Geometry: see drawing. Coordinates: mm, zero at the bounding-box minimum. A direction names the side the tool comes from. Round coordinates to 2 decimals unless told otherwise and drop trailing zeros. Loops run counter-clockwise (first coordinate to the right, second up) from the corner with the lowest first, then second, coordinate; pieces in that order, holes last.
(1) Cut plane C-C, the plane y = 3.75. Output: boundary loops of the cut face in (x, z).
(2) Cut plane D-D, the plane x = 21. Output: boundary loops of the cut face in (y, z), and give its area (3 significant figures).
(3) Cut plane B-B, the plane z = 2.5. Output: boundary loops of the cut face in (x, y), and give its area (3 significant figures).
(4) Cut plane A-A, the plane x = 34. Output: boundary loops of the cut face in (y, z).
(5) Draft query along Y for the marked faces 4, 5 and 6. Return one class per face: released by +Y, released by -Y, zero draft, split by the parting line, or undercut.
(6) Access query for the marked faces 1, 2 and 3. Directions: +Z, -Z, +X, -X, +Y, -Y. A direction counts if a zero-diameter tool reaches every point of the face in a straight line with its end or side. Return the directions, or none.
(7) Line query: line 1 (Y direction, x = 30.5, z = 7.25); line 2 (X direction, y = 2.25, z = 9); line 3 (Y direction, x = 4.5, z = 7.5). Output: solid intervals per line, ascending.
(8) First-contact query: pin 1 Ø5 at (x, z) = (19.5, 5) entering from -Y; pin 2 Ø0.9 at (y, z) = (3.5, 6.5) entering from +X. Flat tips, straight axial feed; report the tip coordinate or a pass-through.
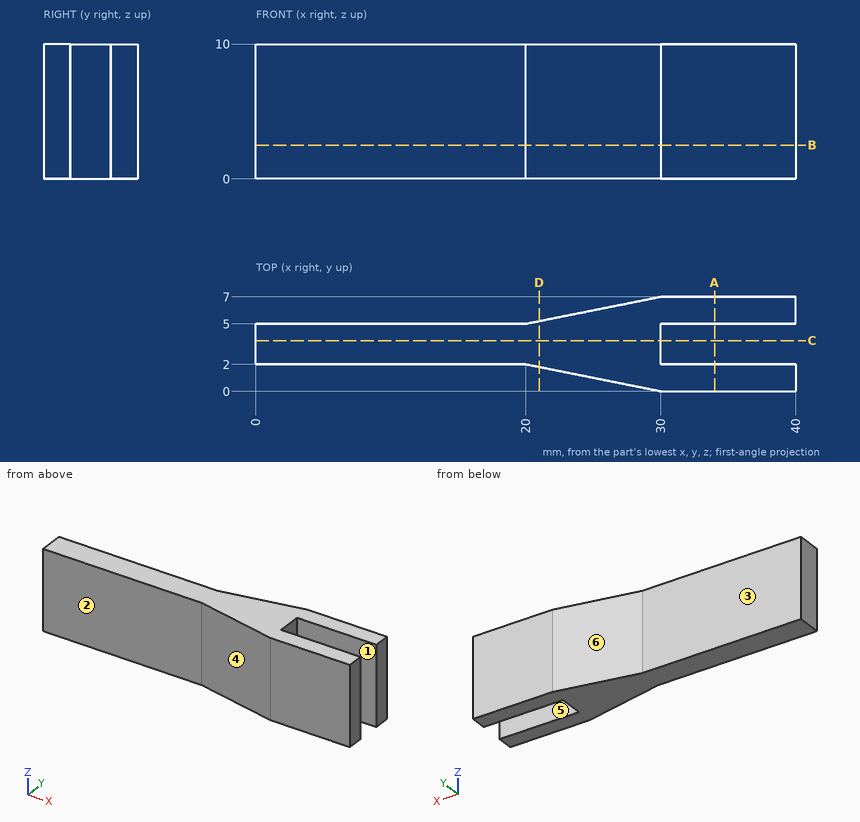
Reported:
1. outline: (0, 0) - (30, 0) - (30, 10) - (0, 10) - close
2. outline: (1.8, 0) - (5.2, 0) - (5.2, 10) - (1.8, 10) - close
2. area: 34.0 mm2
3. outline: (0, 2) - (20, 2) - (30, 0) - (40, 0) - (40, 2) - (30, 2) - (30, 5) - (40, 5) - (40, 7) - (30, 7) - (20, 5) - (0, 5) - close
3. area: 150 mm2
4. outline: (0, 0) - (2, 0) - (2, 10) - (0, 10) - close; (5, 0) - (7, 0) - (7, 10) - (5, 10) - close
5. face 4: released by -Y
5. face 5: undercut
5. face 6: released by +Y
6. face 1: +Z, -Z, +X
6. face 2: +Z, -Z, -X, -Y
6. face 3: +Z, -Z, -X, +Y
7. line 1: y = 0 to 2, 5 to 7
7. line 2: x = 0 to 30
7. line 3: y = 2 to 5
8. pin 1: stops at y = 1.6
8. pin 2: stops at x = 30
